from build123d import *

# Parameters (mm, degrees)
BOSS_EXTRUDE1_DEPTH = 22.86
SKETCH2_W           = 15.494
SKETCH2_H           = 22.86
SKETCH2_R           = 3.2639
BOSS_EXTRUDE2_DEPTH = 5.08
FILLET1_R           = 2.54


with BuildPart() as part:
    # Sketch1 → Boss-Extrude1 (new body)
    with BuildSketch(Plane.XY):
        Polygon((0, 0), (0, -35.052), (72.898, -35.052), (72.898, 0), (76.708, 0), (76.708, -38.862), (-3.81, -38.862), (-3.81, 0), align=None)
    extrude(amount=BOSS_EXTRUDE1_DEPTH)

    # Sketch2 → Boss-Extrude2 (add)
    with BuildSketch(Plane(origin=(0, 0, 0), x_dir=(1, 0, 0), z_dir=(0, 1, 0))):
        with Locations((-7.747, -11.43)):
            Rectangle(SKETCH2_W, SKETCH2_H)
        with Locations(Location((-9.652, -3.81, 0), (0, 0, 270))):
            Circle(SKETCH2_R, mode=Mode.SUBTRACT)
        with Locations(Location((-9.652, -19.05, 0), (0, 0, 270))):
            Circle(SKETCH2_R, mode=Mode.SUBTRACT)
    boss_extrude2 = extrude(amount=-BOSS_EXTRUDE2_DEPTH)

    # Mirror1: Boss-Extrude2 across plane
    add(boss_extrude2.mirror(Plane(origin=(36.449, 0, 0), x_dir=(0, 0, 1), z_dir=(1, 0, 0))))

    # Fillet1
    fillet1_edges = [part.edges().sort_by_distance(p)[0] for p in [
        (-3.81, -5.08, 11.43),
        (76.708, -5.08, 11.43),
    ]]
    fillet(fillet1_edges, radius=FILLET1_R)


solid = part.part
Design review of the part built by this model. Coordinates are the model's own, in mm. A direction names the side the tool comes from. Round coordinates to 2 decimals unless told otherwise and drop trailing zeros. Write each loop counter-clockwise with the first axis right and the second up, starting at its lowest first coordinate (ties: lowest second). Pieces come first, ordered by that corner, then holes.
Item 1: Draft analysis for pull direction X (two halves, no side actions). For faces 1 (the flat face through (-3.81, -23, 11)), 2 (the flat face through (36, -35.052, 11)), 3 (the cylindrical face through (77.472, -5.804, 11.27)), state which applies: released by +X, released by -X, zero draft, split by the parting line, or undercut.
Item 2: For faces 4 (the flat face through (-15.494, -3, 12)), 5 (the flat face through (76.708, -23, 11)), 6 (the flat face through (-12, -5.08, 11)), list the 3-axis set-ups (+Z, -Z, +X, -X, +Y, -Y) from which the entire face can be reached by the end or side of a thin tool; tool diameter is ignored.
Item 3: Wall thickness on L1, parallel to X at y = -2.1, z = 19.05; L2, parallel to Z at x = 82.55, y = -3.7; L3, parallel to X at y = -33, z = 21: over which ranges is each line inside the solid? List them lowest first.
Item 4: Consider section C-C on z = 8. Give the boundary of the cut face in (x, y).
Item 5: Consider section D-D on x = 66. Give the boundary of the cut face in (y, z), and give its area (3 significant figures).
Item 6: For pin 1 Ø7.5 at (x, z) = (-9.652, 19.05) entering from -Y; pin 2 Ø10 at (y, z) = (-32.5, 4) entering from +X; pin 3 Ø8.5 at (x, z) = (82.55, 19.05) entering from -Y, all flat-tipped, find the tip position at first contact; note any pin that passes through.
Item 7: Consider section A-A on y = -24.5. Give the boundary of the cut face in (x, z).
Item 8: Consider section B-B on z = 3.81. Count the separate pieces of the cut face and the enclosed holes in it, and give its area (3 significant figures).
Check values:
1. face 1: released by -X
1. face 2: undercut
1. face 3: released by +X
2. face 4: +Z, -Z, -X, +Y, -Y
2. face 5: +Z, -Z, +X, -Y
2. face 6: +Z, -Z, -X, -Y
3. L1: x = -15.49 to -12.92, -6.39 to 0, 72.9 to 79.29, 85.81 to 88.39
3. L2: z = 0 to 0.55, 7.07 to 15.79, 22.31 to 22.86
3. L3: x = -3.81 to 0, 72.9 to 76.71
4. outline: (-15.49, -5.08) - (-6.35, -5.08) arc R2.54 cw to (-3.81, -7.62) - (-3.81, -38.86) - (76.71, -38.86) - (76.71, -7.62) arc R2.54 cw to (79.25, -5.08) - (88.39, -5.08) - (88.39, 0) - (72.9, 0) - (72.9, -35.05) - (0, -35.05) - (0, 0) - (-15.49, 0) - close
5. outline: (-38.86, 0) - (-35.05, 0) - (-35.05, 22.86) - (-38.86, 22.86) - close
5. area: 87.1 mm2
6. pin 1: stops at y = -5.12
6. pin 2: stops at x = 76.71
6. pin 3: stops at y = -5.26
7. outline: (-3.81, 0) - (0, 0) - (0, 22.86) - (-3.81, 22.86) - close; (72.9, 0) - (76.71, 0) - (76.71, 22.86) - (72.9, 22.86) - close
8. separate pieces: 3
8. enclosed holes: 0
8. area: 629 mm2
